```python
from build123d import *

# Parameters (mm, degrees)
SKETCH1_R           = 42.5
SKETCH1_R_2         = 33
BOSS_EXTRUDE1_DEPTH = 10
SKETCH2_R           = 2.25
CUT_EXTRUDE1_DEPTH  = 11
CIRPATTERN1_COUNT   = 12
SKETCH3_R           = 2.25
CUT_EXTRUDE2_DEPTH  = 11
CIRPATTERN2_COUNT   = 2


with BuildPart() as part:
    # Sketch1 → Boss-Extrude1 (new body)
    with BuildSketch(Plane(origin=(0, 0, 0), x_dir=(1, 0, 0), z_dir=(0, 1, 0))):
        Circle(SKETCH1_R)
        Circle(SKETCH1_R_2, mode=Mode.SUBTRACT)
    extrude(amount=BOSS_EXTRUDE1_DEPTH)

    # Sketch2 → Cut-Extrude1 (cut, through all)
    with BuildSketch(Plane(origin=(0, 10, 0), x_dir=(1, 0, 0), z_dir=(0, 1, 0))):
        with Locations((0, 37.5)):
            Circle(SKETCH2_R)
    cut_extrude1 = extrude(amount=-CUT_EXTRUDE1_DEPTH, mode=Mode.SUBTRACT)

    # CirPattern1: Cut-Extrude1 ×12 about axis
    cirpattern1_axis = Axis((0, 0, 0), (0, 1, 0))
    for i in range(1, CIRPATTERN1_COUNT):
        add(cut_extrude1.rotate(cirpattern1_axis, i * 360 / CIRPATTERN1_COUNT), mode=Mode.SUBTRACT)

    # Sketch3 → Cut-Extrude2 (cut, through all)
    with BuildSketch(Plane(origin=(0, 10, 0), x_dir=(1, 0, 0), z_dir=(0, 1, 0))):
        with Locations((-9.705714191, 36.222218486)):
            Circle(SKETCH3_R)
    cut_extrude2 = extrude(amount=-CUT_EXTRUDE2_DEPTH, mode=Mode.SUBTRACT)

    # CirPattern2: Cut-Extrude2 ×2 about axis
    cirpattern2_axis = Axis((0, 0, 0), (0, 1, 0))
    for i in range(1, CIRPATTERN2_COUNT):
        add(cut_extrude2.rotate(cirpattern2_axis, i * 360 / CIRPATTERN2_COUNT), mode=Mode.SUBTRACT)


solid = part.part
```
Read the model definition and answer for the solid it produces. Units are mm, in the model's axes. Coordinates: 2 decimals unless noted, no trailing zeros. Write each loop counter-clockwise with the first axis right and the second up, starting at its lowest first coordinate (ties: lowest second). Pieces come first, ordered by that corner, then holes. Notation, with made-up numbers: (83, 48) -> (90, 48) arc R19 cw to (90, 57) -> close; hole circle Ø11 at (-34, -15.5). An arc over 180 degrees is marked (long way). Write item = value, one per line.
(1) Section B-B on z = 18 is taken. Write down the section's boundary in (x, y), plus the area to 3 significant figures.
From the geometry:
outline = (-38.5, 0) -> (-34.6, 0) -> (-34.6, 10) -> (-38.5, 10) -> close; (-30.35, 0) -> (-27.66, 0) -> (-27.66, 10) -> (-30.35, 10) -> close; (27.66, 0) -> (30.35, 0) -> (30.35, 10) -> (27.66, 10) -> close; (34.6, 0) -> (38.5, 0) -> (38.5, 10) -> (34.6, 10) -> close
area = 132 mm2
(2) Given pin 1 Ø1.5 at (x, y) = (33, 3) entering from +Z; pin 2 Ø6 at (x, y) = (32.5, 3.5) entering from +Z; pin 3 Ø3 at (y, z) = (3.5, -29.5) entering from -X, each flat-ended and moving along its own axis, determine where each tip first touches the part or whether it passes through.
From the geometry:
pin_1 = 27.68
pin_2 = 30.59
pin_3 = -31.97
(3) Section C-C on z = -37.5 is taken. Write down the section's boundary in (x, y).
From the geometry:
outline = (-20, 0) -> (-11.56, 0) -> (-11.56, 10) -> (-20, 10) -> close; (-7.85, 0) -> (-2.25, 0) -> (-2.25, 10) -> (-7.85, 10) -> close; (2.25, 0) -> (20, 0) -> (20, 10) -> (2.25, 10) -> close
(4) Straight lines are drawn through the part: L1, parallel to Z at x = 0, y = 6.5; L2, parallel to Z at x = 17.5, y = 1; L3, parallel to Z at x = -34, y = 9.25. For each, find the intervals that lie inside material, in ascending order. Write a range as from..to.
From the geometry:
L1 = -42.5..-39.75, -35.25..-33, 33..35.25, 39.75..42.5
L2 = -38.73..-34.35, -30.61..-27.98, 27.98..30.61, 34.35..38.73
L3 = -25.5..-20.41, -17.09..17.09, 20.41..25.5
(5) Section A-A on x = -37.5 is taken. Write down the section's boundary in (y, z), plus the area to 3 significant figures.
From the geometry:
outline = (0, -20) -> (10, -20) -> (10, -2.25) -> (0, -2.25) -> close; (0, 2.25) -> (10, 2.25) -> (10, 20) -> (0, 20) -> close
area = 355 mm2
(6) For a pull along Z with two mould halves and no side action, classify faces 1 (the face through (-17.229, 5.07, -34.134)), 2 (the face through (-10, 0, -32)), 3 (the face through (-33.727, 4.93, 25.861)), 4 (the face through (-0.29, 5.07, -39.73)) as +Z half, -Z half, draft (parallel to the pull), parting line (faces both ways), or undercut.
From the geometry:
face_1 = undercut
face_2 = draft
face_3 = parting line
face_4 = undercut
(7) Section D-D on x = -18.75 is taken. Write down the section's boundary in (y, z).
From the geometry:
outline = (0, -38.14) -> (10, -38.14) -> (10, -34.73) -> (0, -34.73) -> close; (0, -30.23) -> (10, -30.23) -> (10, -27.16) -> (0, -27.16) -> close; (0, 27.16) -> (10, 27.16) -> (10, 30.23) -> (0, 30.23) -> close; (0, 34.73) -> (10, 34.73) -> (10, 38.14) -> (0, 38.14) -> close
